Autodesk Inventor part; units mm, degrees
ref_plane "YZ Plane" through (0, 0, 0) normal (1, 0, 0) x (0, 1, 0)
ref_plane "XZ Plane" through (0, 0, 0) normal (0, 1, 0) x (-1, 0, 0)
ref_plane "XY Plane" through (0, 0, 0) normal (0, 0, 1) x (1, 0, 0)
sketch "Sketch1" plane through (0, 0, 0) normal (0, 1, 0) x (-1, 0, 0)
  line L0 (-45, 125) -> (45, 125)
  line L1 (45, 125) -> (45, -125)
  line L2 (45, -125) -> (-45, -125)
  line L3 (-45, -125) -> (-45, 125)
  line L4 (-45, 125) -> (45, -125) construction
  line L5 (45, 125) -> (-45, -125) construction
  point P0 (0, 0)
  dimension "d0" = 250
  dimension "d1" = 90
extrude "Extrusion1" add sketch "Sketch1" along normal blind 10
sketch "Sketch2" plane through (-45, 0, 125) normal (0, 0, 1) x (1, 0, 0)
  line L0 (90, 10) -> (0, 10)
  line L1 (0, 10) -> (90, 10)
  line L2 (90, 10) -> (90, 50)
  line L3 (90, 50) -> (0, 50)
  line L4 (0, 50) -> (0, 10)
  point P0 (45, 0)
  dimension "d4" = 40
extrude "Extrusion2" add sketch "Sketch2" against normal blind 10
sketch "Sketch3" plane through (45, 0, -125) normal (0, 0, -1) x (-1, 0, 0)
  line L0 (0, 0) -> (0, 50)
  line L1 (90, 0) -> (90, 50)
  line L2 (0, 9.2486) -> (90, 9.2486)
  line L3 (90, 9.2486) -> (90, 50)
  line L4 (90, 50) -> (0, 50)
  line L5 (0, 50) -> (0, 9.2486)
  point P0 (45, 0)
  point P1 (90, 9.2486)
extrude "Extrusion3" cut sketch "Sketch3" against normal blind 10
sketch "Sketch4" plane through (45, 0, -125) normal (0, 0, -1) x (-1, 0, 0)
  line L0 (90, 10) -> (0, 10)
  line L1 (90, 10) -> (90, 50)
  line L2 (0, 10) -> (90, 10)
  line L3 (90, 10) -> (90, 50)
  line L4 (90, 50) -> (0, 50)
  line L5 (0, 50) -> (0, 10)
  point P0 (45, 0)
extrude "Extrusion4" add sketch "Sketch4" against normal blind 10
sketch "Sketch5" plane through (-45, 0, -125) normal (-1, 0, 0) x (0, 0, 1)
  line L0 (10, 50) -> (10, 10)
  line L1 (240, 50) -> (240, 10)
  line L2 (10, 10) -> (240, 10)
  line L3 (240, 10) -> (240, 50)
  line L4 (240, 50) -> (10, 50)
  line L5 (10, 50) -> (10, 10)
  point P0 (125, 0)
extrude "Extrusion5" add sketch "Sketch5" against normal blind 10
properties part number "aaa"
Source: CAD feature listing. Evaluate the final solid. Frame: model axes, mm. A direction names the side the tool comes from. Give positions to 0.01 mm unless a question says otherwise; leave off trailing zeros. Loops run counter-clockwise (first coordinate to the right, second up) from the corner with the lowest first, then second, coordinate; pieces in that order, holes last. Notation, with made-up numbers: (13.5, 34) -> (54.5, 34) arc R23 ccw to (54.5, 58) -> close; hole circle Ø5 at (-13, 2). An arc over 180 degrees is marked (long way). Put each result on its own line as item: value. Start each with the question number.
1) Cut plane B-B (y = 38.5). Return loops of the section in (x, z), then the cut area to 3 significant figures.
2) Draft query along Z for faces 1 (the face through (-1, 10, -120)), 2 (the face through (-1, 5, -125)), 3 (the face through (4, 30, 115)). Return one class per face: released by +Z, released by -Z, zero draft, split by the parting line, or undercut.
3) Reachability of faces 4 (the face through (1, 30, -125)), 5 (the face through (6, 30, -115)), 6 (the face through (1, 9.249, -120)) from +Z, -Z, +X, -X, +Y, -Y: full face, straight path, thin tool, end or side. Return the list, or none.
4) Contact query for flat-ended pins moving along their axis: P1, Ø8, axis at y = 31, z = 57.5, coming from the +X side; P2, Ø1, axis at x = -17.5, z = -20.5, coming from the +Y side. Output: stop coordinate, or through.
5) Material intervals for probe 1 along Z at (x, y) = (24, 37.5); probe 2 along Y at (x, z) = (-28, -11); probe 3 along X at (y, z) = (43, 84), sorted ascending.
6) Cut plane C-C (z = -82). Return loops of the section in (x, y), then the cut area to 3 significant figures.
Results are:
1. outline: (-45, -125) -> (45, -125) -> (45, -115) -> (-35, -115) -> (-35, 115) -> (45, 115) -> (45, 125) -> (-45, 125) -> close
1. area: 4,100 mm2
2. face 1: zero draft
2. face 2: released by -Z
2. face 3: undercut
3. face 4: -Z, +X, -X, +Y, -Y
3. face 5: +X, +Y
3. face 6: -Z, +X, -X
4. P1: stops at x = -35
4. P2: stops at y = 10
5. probe 1: z = -125 to -115, 115 to 125
5. probe 2: y = 0 to 10
5. probe 3: x = -45 to -35
6. outline: (-45, 0) -> (45, 0) -> (45, 10) -> (-35, 10) -> (-35, 50) -> (-45, 50) -> close
6. area: 1,300 mm2
